Source: CAD feature listing. Evaluate the final solid. Frame: model axes, mm. A direction names the side the tool comes from. Round coordinates to 2 decimals unless told otherwise and drop trailing zeros. Write each loop counter-clockwise with the first axis right and the second up, starting at its lowest first coordinate (ties: lowest second). Pieces come first, ordered by that corner, then holes. Notation, with made-up numbers: M 22,-19.75 L 49,-19.75 A22 cw 49,-13.75 Z; hole C -35.75,64 d11. An arc over 180 degrees is marked long. Answer in a Markdown table with one row per item. Add a question column.
Item 1: Material intervals for probe 1 along Z at (x, y) = (0.5, 3.5), sorted ascending.
Item 2: Contact query for flat-ended pins moving along their axis: pin 1 (6 mm diameter, centred on x = -3, y = 127, fed in from -Z); pin 2 (7.5 mm diameter, centred on x = -4.5, y = -71, fed in from +Z); pin 3 (7.5 mm diameter, centred on x = 7.5, z = -169, fed in from -Y) (3 decimals). Output: stop coordinate, or through.
Item 3: Cut plane A-A on y = -95.5. Return loops of the section in (x, z) (3 decimals).
Item 4: Set-up query: faces 1 (the face through (3.175, 12, -171)), 2 (the face through (8, 161.925, 171)), 3 (the face through (8, 161.925, -171)), 4 (the face through (8, -142.875, 171)). Return all of +Z, -Z, +X, -X, +Y, -Y with unobstructed straight access to the full face (end or side cutting, diameter ignored); none if empty.
Item 5: Cut plane B-B on x = -8. Return loops of the section in (y, z) (3 decimals), and give its area (3 significant figures).
from build123d import *

# Parameters (mm, degrees)
F0_W     = 349.25
F0_H     = 328.6125
F1_DEPTH = 12.7
F2_W     = 9.525
F2_H     = 304.8
F3_DEPTH = 12.7
F4_W     = 9.525
F4_H     = 304.8
F5_DEPTH = 12.7


with BuildPart() as f1:
    # F0 (on Right) → F1 (new body, symmetric)
    with BuildSketch(Plane.YZ):
        Rectangle(F0_W, F0_H)
    extrude(amount=F1_DEPTH, both=True)

    # F2 (on face) → F3 (join)
    with BuildSketch(Plane.XY.offset(164.30625)):
        with Locations((7.9375, 9.525)):
            Rectangle(F2_W, F2_H)
    extrude(amount=F3_DEPTH)

    # F4 (on face) → F5 (join)
    with BuildSketch(Plane(origin=(0, 0, -164.30625), x_dir=(1, 0, 0), z_dir=(0, 0, -1))):
        with Locations((7.9375, -9.525)):
            Rectangle(F4_W, F4_H)
    extrude(amount=F5_DEPTH)


solid = f1.part
Results below:
| question | item | result |
|---|---|---|
| 1 | probe 1 | -164.31 to 164.31 |
| 2 | pin 1 | z = -164.31 |
| 2 | pin 2 | z = 164.31 |
| 2 | pin 3 | y = -142.875 |
| 3 | outline | M -12.7,-164.306 L 3.175,-164.306 L 3.175,-177.006 L 12.7,-177.006 L 12.7,177.006 L 3.175,177.006 L 3.175,164.306 L -12.7,164.306 Z |
| 4 | face 1 | -Z, -X, +Y, -Y |
| 4 | face 2 | +Z, +X, -X, +Y |
| 4 | face 3 | -Z, +X, -X, +Y |
| 4 | face 4 | +Z, +X, -X, -Y |
| 5 | outline | M -174.625,-164.306 L 174.625,-164.306 L 174.625,164.306 L -174.625,164.306 Z |
| 5 | area | 115,000 mm2 |
